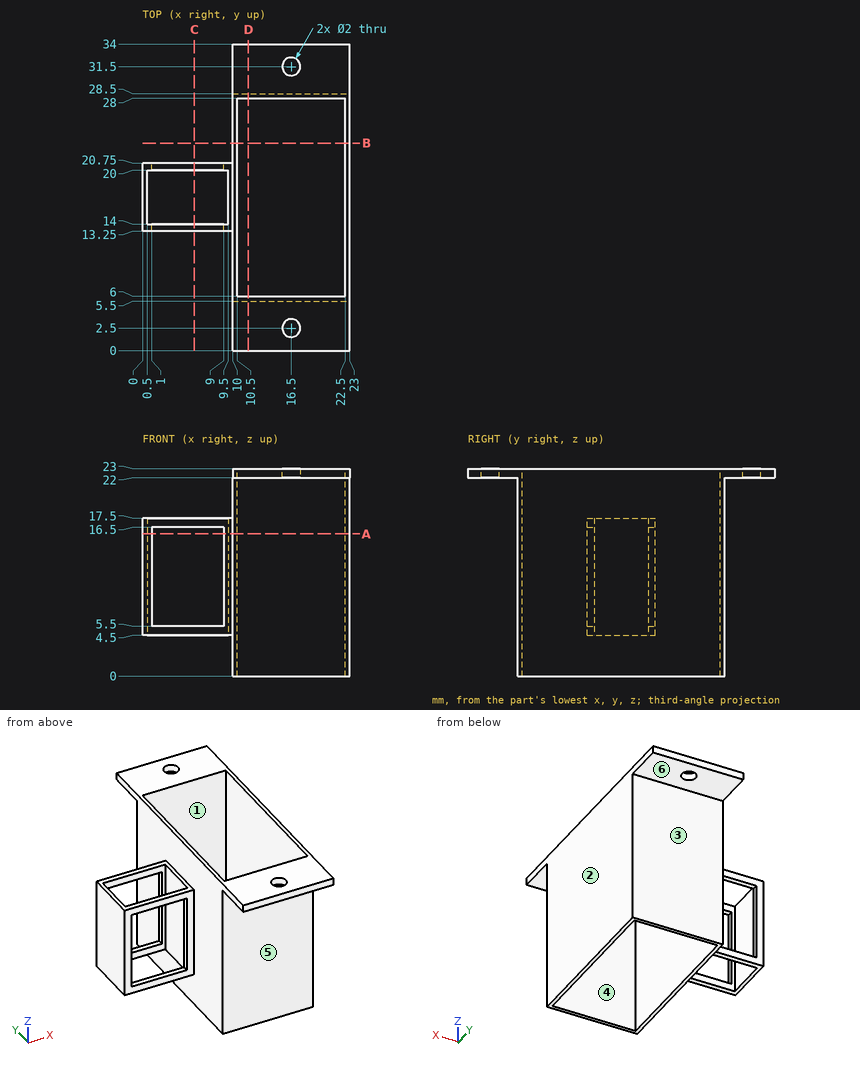
Input: dimensioned drawing with shaded views. Units: mm. Origin: part minimum x, y, z. A direction names the side the tool comes from. Round coordinates to 2 decimals unless told otherwise and drop trailing zeros. Order: outer loops, then holes, each group sorted by start corner. A loop starts at its lowest first (then second) coordinate and runs counter-clockwise, first axis right, second up.
1. Set-up query: the marked faces 1, 2 and 3. Return all of +Z, -Z, +X, -X, +Y, -Y with unobstructed straight access to the full face (end or side cutting, diameter ignored); none if empty.
The answers:
face 1: +Z, -Z
face 2: +Z, -Z, +X, +Y, -Y
face 3: -Z, +X, -X, +Y
2. Pin query (flat end, axial travel): P1, Ø6, axis at x = 14.5, y = 18.5, coming from the -Z side; P2, Ø1.5, axis at x = 15.5, z = 20, coming from the +Y side; P3, Ø4, axis at x = 4, y = 18.5, coming from the +Z side; P4, Ø9.5, axis at x = 14, z = 13.5, coming from the -Y side. Return the tip coordinate at first contact, or that it passes through.
The answers:
P1: passes through
P2: stops at y = 28.5
P3: stops at z = 17.5
P4: stops at y = 5.5
3. Cut plane C-C, the plane x = 5.75. Output: boundary loops of the cut face in (y, z), then the cut area to 3 significant figures.
The answers:
outline: (13.25, 4.5) - (14, 4.5) - (14, 5.5) - (13.25, 5.5) - close; (13.25, 16.5) - (14, 16.5) - (14, 17.5) - (13.25, 17.5) - close; (20, 4.5) - (20.75, 4.5) - (20.75, 5.5) - (20, 5.5) - close; (20, 16.5) - (20.75, 16.5) - (20.75, 17.5) - (20, 17.5) - close
area: 3.00 mm2
4. Material intervals for line 1 (Y direction, x = 16.5, z = 22.7); line 2 (X direction, y = 10, z = 14.75); line 3 (Y direction, x = 19.25, z = 15.75), sorted ascending.
The answers:
line 1: y = 0 to 1.5, 3.5 to 6, 28 to 30.5, 32.5 to 34
line 2: x = 10 to 10.5, 22.5 to 23
line 3: y = 5.5 to 6, 28 to 28.5
5. Cut plane B-B, the plane y = 23. Output: boundary loops of the cut face in (x, z).
The answers:
outline: (10, 0) - (10.5, 0) - (10.5, 23) - (10, 23) - close; (22.5, 0) - (23, 0) - (23, 23) - (22.5, 23) - close
6. Cut plane A-A, the plane z = 15.75. Output: boundary loops of the cut face in (x, y), then the cut area to 3 significant figures.
The answers:
outline: (0, 13.25) - (1, 13.25) - (1, 14) - (0.5, 14) - (0.5, 20) - (1, 20) - (1, 20.75) - (0, 20.75) - close; (9, 13.25) - (10, 13.25) - (10, 5.5) - (23, 5.5) - (23, 28.5) - (10, 28.5) - (10, 20.75) - (9, 20.75) - (9, 20) - (9.5, 20) - (9.5, 14) - (9, 14) - close; hole (10.5, 6) - (22.5, 6) - (22.5, 28) - (10.5, 28) - close
area: 44.0 mm2
7. Mould query, pull axis Y, two halves, no side actions, for the marked faces 4, 5 and 6. Classes: released by +Y, released by -Y, zero draft, split by the parting line, or undercut.
The answers:
face 4: undercut
face 5: released by -Y
face 6: zero draft
8. Cut plane D-D, the plane x = 11.75. Output: boundary loops of the cut face in (y, z).
The answers:
outline: (0, 22) - (5.5, 22) - (5.5, 0) - (6, 0) - (6, 23) - (0, 23) - close; (28, 0) - (28.5, 0) - (28.5, 22) - (34, 22) - (34, 23) - (28, 23) - close
